Geometry check sheet. Reference: drawing and pictorial views, mm from the part's lowest x, y, z. Give positions to 0.01 mm unless a question says otherwise; leave off trailing zeros. Loops run counter-clockwise (first coordinate to the right, second up) from the corner with the lowest first, then second, coordinate; pieces in that order, holes last. Notation, with made-up numbers: (2.5, 25) - (60.5, 25) arc R20 cw to (60.5, 58) - close; hole circle Ø7 at (25.25, -33.5). An arc over 180 degrees is marked (long way). One line per question, with ' | ' between items. Start each with the question number.
1. Thickness scan on line 1 along X through (y, z) = (30, 10); line 2 along Y through (x, z) = (203, 12); line 3 along X through (y, z) = (19, 28). Record the ranges inside material, lowest first. Write a range as from..to.
2. Section check B-B, the plane x = 203. Enter the section's corners in (y, z), then the cut area to 3 significant figures.
3. Section check D-D, the plane z = 36.5. Enter the section's corners in (x, y), then the cut area to 3 significant figures.
4. Depth check by flat-ended pin: pin 1 Ø3 at (x, y) = (203, 90) entering from -Z. Enter the tip coordinate at first touch or a pass-through.
5. Section check A-A, the plane z = 6. Enter the section's corners in (x, y).
6. Section check C-C, the plane y = 90. Enter the section's corners in (x, z), then the cut area to 3 significant figures.
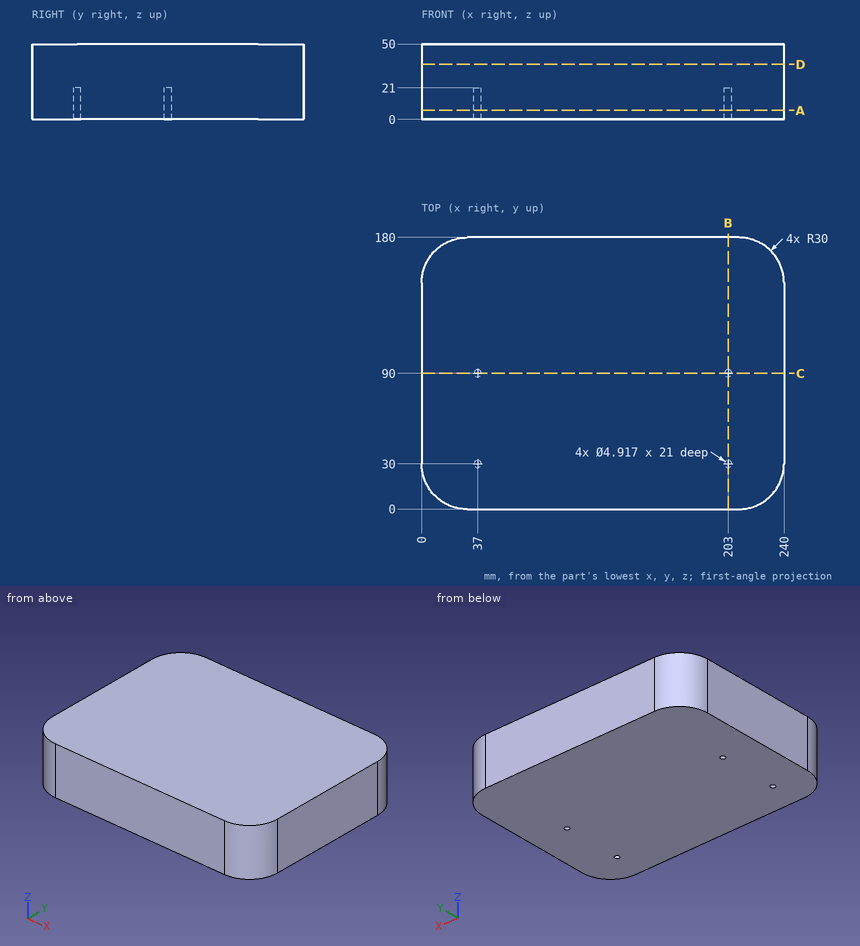
Results list:
1) line 1: 0..34.54, 39.46..200.54, 205.46..240 | line 2: 0..27.54, 32.46..87.54, 92.46..180 | line 3: 2.09..237.91
2) outline: (0, 0) - (27.54, 0) - (27.54, 21) - (32.46, 21) - (32.46, 0) - (87.54, 0) - (87.54, 21) - (92.46, 21) - (92.46, 0) - (180, 0) - (180, 50) - (0, 50) - close | area: 8,790 mm²
3) outline: (0, 30) arc R30 ccw to (30, 0) - (210, 0) arc R30 ccw to (240, 30) - (240, 150) arc R30 ccw to (210, 180) - (30, 180) arc R30 ccw to (0, 150) - close | area: 42,400 mm²
4) pin 1: z = 21
5) outline: (0, 30) arc R30 ccw to (30, 0) - (210, 0) arc R30 ccw to (240, 30) - (240, 150) arc R30 ccw to (210, 180) - (30, 180) arc R30 ccw to (0, 150) - close; hole circle Ø4.92 at (37, 30); hole circle Ø4.92 at (37, 90); hole circle Ø4.92 at (203, 30); hole circle Ø4.92 at (203, 90)
6) outline: (0, 0) - (34.54, 0) - (34.54, 21) - (39.46, 21) - (39.46, 0) - (200.54, 0) - (200.54, 21) - (205.46, 21) - (205.46, 0) - (240, 0) - (240, 50) - (0, 50) - close | area: 11,800 mm²
